from build123d import *

# Parameters (mm, degrees)
F0_R     = 2.55
F1_DEPTH = 1600.2


with BuildPart() as f1:
    # F0 (on Top) → F1 (new body)
    with BuildSketch(Plane.XY):
        with BuildLine():
            ThreePointArc((4.241495, 5.404315), (3.435, 5.949595), (2.559526, 6.3754))
            Line((2.559526, 6.3754), (-2.559526, 6.3754))
            ThreePointArc((-2.559526, 6.3754), (-3.435, 5.949595), (-4.241495, 5.404315))
            Line((-4.241495, 5.404315), (-6.801022, 0.971085))
            ThreePointArc((-6.801022, 0.971085), (-6.87, 0), (-6.801022, -0.971085))
            Line((-6.801022, -0.971085), (-4.241495, -5.404315))
            ThreePointArc((-4.241495, -5.404315), (-3.435, -5.949595), (-2.559526, -6.3754))
            Line((-2.559526, -6.3754), (2.559526, -6.3754))
            ThreePointArc((2.559526, -6.3754), (3.435, -5.949595), (4.241495, -5.404315))
            Line((4.241495, -5.404315), (6.801022, -0.971085))
            ThreePointArc((6.801022, -0.971085), (6.87, 0), (6.801022, 0.971085))
            Line((6.801022, 0.971085), (4.241495, 5.404315))
        make_face()
        Circle(F0_R, mode=Mode.SUBTRACT)
    extrude(amount=F1_DEPTH)


solid = f1.part
Source: CAD feature listing. Evaluate the final solid. Frame: model axes, mm. Round coordinates to 2 decimals unless told otherwise and drop trailing zeros. Order: outer loops, then holes, each group sorted by start corner. A loop starts at its lowest first (then second) coordinate and runs counter-clockwise, first axis right, second up. Notation, with made-up numbers: (65.25, 51) - (95.25, 51) arc R32 ccw to (95.25, 85) - close; hole circle Ø10 at (-9, 43). An arc over 180 degrees is marked (long way). Use a Markdown table: item, result. Add a question column.
1. First-contact query: pin 1 (1.5 mm diameter, centred on x = 2.5, y = -0.5, fed in from -Z); pin 2 (4 mm diameter, centred on x = -5, z = 624.5, fed in from +Y); pin 3 (1.5 mm diameter, centred on y = 1.5, z = 1202.5, fed in from +X). Flat tips, straight axial feed; report the tip coordinate or a pass-through.
2. Section query B-B (z = 376.5). Return the cut outline in (x, y).
3. Line query: probe 1 along Y at (x, z) = (-1, 1459); probe 2 along Y at (x, z) = (0, 1109.5); probe 3 along X at (y, z) = (-0.75, 539). Output: solid intervals per line, ascending.
4. Section query A-A (x = 0). Return the cut outline in (y, z), then the cut area to 3 significant figures.
Derived:
| question | item | result |
|---|---|---|
| 1 | pin 1 | z = 0 |
| 1 | pin 2 | y = 6.18 |
| 1 | pin 3 | x = 6.83 |
| 2 | outline | (-6.8, -0.97) - (-4.24, -5.4) arc R6.87 ccw to (-2.56, -6.38) - (2.56, -6.38) arc R6.87 ccw to (4.24, -5.4) - (6.8, -0.97) arc R6.87 ccw to (6.8, 0.97) - (4.24, 5.4) arc R6.87 ccw to (2.56, 6.38) - (-2.56, 6.38) arc R6.87 ccw to (-4.24, 5.4) - (-6.8, 0.97) arc R6.87 ccw to start; hole circle Ø5.1 at (0, 0) |
| 3 | probe 1 | -6.38 to -2.35, 2.35 to 6.38 |
| 3 | probe 2 | -6.38 to -2.55, 2.55 to 6.38 |
| 3 | probe 3 | -6.83 to -2.44, 2.44 to 6.83 |
| 4 | outline | (-6.38, 0) - (-2.55, 0) - (-2.55, 1600.2) - (-6.38, 1600.2) - close; (2.55, 0) - (6.38, 0) - (6.38, 1600.2) - (2.55, 1600.2) - close |
| 4 | area | 12,200 mm2 |
